Build history of the part. All positions in model axes, mm. A direction names the side the tool comes from. Round coordinates to 2 decimals unless told otherwise and drop trailing zeros. Loops run counter-clockwise (first coordinate to the right, second up) from the corner with the lowest first, then second, coordinate; pieces in that order, holes last. Notation, with made-up numbers: (-33.5, -16) - (-22.5, -16) arc R10 cw to (-22.5, 1) - close; hole circle Ø7 at (9, 10.5). An arc over 180 degrees is marked (long way). Use one line per item in the form item = value. Start each with the question number.
Q1. Pin check, flat tips, straight feed: pin 1 (3 mm diameter, centred on y = 4.5, z = -0.5, fed in from +X); pin 2 (4.5 mm diameter, centred on x = 5.5, z = 2, fed in from +Y); pin 3 (1.5 mm diameter, centred on x = 9.5, y = 6, fed in from -Z); pin 4 (1.8 mm diameter, centred on x = 5.5, y = 4, fed in from +Z). Stop position of each tip, or through.
Q2. Saw through at C-C (y = 2). Give the cut face in (x, z).
Q3. Saw through at A-A (x = 6). Give the cut face in (y, z) (3 decimals), then the cut area to 3 significant figures.
Q4. Saw through at B-B (z = 3). Give the cut face in (x, y) (3 decimals).
Q5. Drill centre lines: line 1 (Y direction, x = 38, z = 3) (3 decimals); line 2 (Y direction, x = 6, z = 5.3); line 3 (X direction, y = 10.5, z = -5). Where is each one in solid material? Low to high.
Q6. Mould opens along X. For faces 6 (the face through (0, 4, 3)), 7 (the face through (38, 6.5, 0.15)), 8 (the face through (6, 2, 4)), 9 (the face through (35, 4.6, 5)) say: released by +X, released by -X, zero draft, split by the parting line, or undercut.
Q7. Saw through at D-D (z = 5). Give the cut face in (x, y), then the cut area to 3 significant figures.
Q8. 3-axis set-ups, long thin cutter, end or side, ignore diameter. For faces 1 (the face through (6, 8.85, 3)), 2 (the face through (38, 8.85, 3)), 3 (the face through (8, 5, 0.15)), 4 (the face through (22, 5, 6)), 5 (the face through (40, 5, 4)): which of +Z, -Z, +X, -X, +Y, -Y reach the whole face in a straight line?
Autodesk Inventor part; units mm, degrees
ref_plane "YZ Plane" through (0, 0, 0) normal (1, 0, 0) x (0, 1, 0)
ref_plane "XZ Plane" through (0, 0, 0) normal (0, 1, 0) x (-1, 0, 0)
ref_plane "XY Plane" through (0, 0, 0) normal (0, 0, 1) x (1, 0, 0)
sketch "Sketch1" plane through (0, 0, 0) normal (0, 0, 1) x (1, 0, 0)
  line L0 (0, 0) -> (44, 0)
  line L1 (44, 0) -> (44, 8.85)
  line L2 (31.85, 12) -> (12.15, 12)
  line L3 (0, 8.85) -> (0, 0)
  line L4 (12.15, 12) -> (12.15, 8.85)
  line L5 (12.15, 8.85) -> (0, 8.85)
  line L6 (31.85, 12) -> (31.85, 8.85)
  line L7 (31.85, 8.85) -> (44, 8.85)
  dimension "d6" = 44
  dimension "d7" = 3.15
  dimension "d8" = 3.15
  dimension "d9" = 12.15
  dimension "d10" = 12.15
  dimension "d11" = 8.85
  dimension "d12" = 8.85
  dimension "d13" = 12
extrude "Extrusion1" add sketch "Sketch1" along normal blind 6
sketch "Sketch2" plane through (0, 0, 0) normal (0, 0, -1) x (-1, 0, 0)
  line L0 (-31.85, 12) -> (-12.15, 12)
  line L1 (0, 0) -> (-44, 0)
  line L2 (-31.85, 12) -> (-12, 12)
  line L3 (-12, 12) -> (-12, 0)
  line L4 (-12, 0) -> (-31.85, 0)
  line L5 (-31.85, 0) -> (-31.85, 12)
extrude "Extrusion2" add sketch "Sketch2" along normal blind 6
sketch "Sketch3" plane through (0, 0, 0) normal (0, 0, -1) x (-1, 0, 0)
  circle A0 centre (-6, 4.35) radius 1.725
  line L0 (-12, 8.85) -> (0, 8.85)
  line L1 (0, 8.85) -> (0, 0)
  circle A1 centre (-38, 4.5) radius 1.725
  line L2 (-31.85, 0) -> (-44, 0)
  line L3 (-44, 0) -> (-44, 8.85)
  point P0 (-12, 9)
  dimension "d18" = 3.45
  dimension "d19" = 4.5
  dimension "d20" = 6
  dimension "d21" = 3.45
  dimension "d22" = 4.5
  dimension "d23" = 6
extrude "Extrusion3" cut sketch "Sketch3" against normal blind 4
sketch "Sketch4" plane through (0, 0, 6) normal (0, 0, 1) x (1, 0, 0)
  circle A0 centre (6, 4.35) radius 3
  line L0 (12.15, 8.85) -> (0, 8.85)
  line L1 (0, 8.85) -> (0, 0)
  circle A1 centre (38, 4.5) radius 1.725
  circle A2 centre (38, 4.5) radius 3
  dimension "d26" = 6
  dimension "d27" = 4.5
  dimension "d28" = 6
  dimension "d29" = 6
extrude "Extrusion4" cut sketch "Sketch4" against normal blind 2 contours A0 | A1 | A2
sketch "Sketch5" plane through (31.85, 0, 0) normal (0, -1, 0) x (1, 0, 0)
  point P0 (-31.85, 0)
sketch "Sketch6" plane through (0, 0, 0) normal (0, 0, -1) x (-1, 0, 0)
  line L0 (0, 0) -> (-44, 0)
  line L1 (-12.15, 8.85) -> (0, 8.85)
  line L2 (0, 0) -> (0, 8.85)
  line L3 (-12.15, 8.85) -> (-12, 8.85)
  line L4 (0, 8.85) -> (-12, 8.85)
  line L5 (-12, 0) -> (-12, 12)
  line L6 (-12, 8.85) -> (-12, 0)
  line L7 (-12, 0) -> (0, 0)
  line L8 (-44, 0) -> (-44, 8.85)
  line L9 (-44, 0) -> (-31.85, 0)
  line L10 (-31.85, 0) -> (-31.85, 8.85)
  line L11 (-31.85, 0) -> (-31.85, 8.85)
  line L12 (-31.85, 8.85) -> (-44, 8.85)
  line L13 (-44, 8.85) -> (-44, 0)
  dimension "d33" = 12.15
extrude "Extrusion5" cut sketch "Sketch6" against normal blind 0.15
sketch "Sketch7" plane through (12, 8.85, 0) normal (-1, 0, 0) x (0, 0, 1)
  line L0 (0, 3.15) -> (0, 0)
  line L1 (0, 3.15) -> (0, 0)
  line L2 (0.15, 0) -> (6, 0)
  line L3 (0, 0) -> (0.15, 0)
  line L4 (0.15, 0) -> (0.15, -8.85)
  line L5 (0.15, 0) -> (0.15, -8.85)
  line L6 (0.15, -8.85) -> (-6, -8.85)
  line L7 (0.15, -8.85) -> (-6, -8.85)
  line L8 (-6, -8.85) -> (-6, 3.15)
  line L9 (0, 3.15) -> (6, 3.15)
  line L10 (-6, 3.15) -> (0, 3.15)
  point P0 (0, -8.85)
sketch "Sketch8" plane through (12.15, 12, 6) normal (0, 1, 0) x (1, 0, 0)
  line L0 (0, 6) -> (0, 0)
  line L1 (19.7, 12) -> (-0.15, 12)
  line L2 (0, 6) -> (-0.15, 6)
  line L3 (-0.15, 6) -> (-0.15, 12)
  line L4 (-0.15, 12) -> (0, 12)
  line L5 (0, 12) -> (0, 6)
  point P0 (-12.15, 6)
extrude "Extrusion6" cut sketch "Sketch7" against normal blind 0.15
fillet "Fillet2" radius 1.5 2 edges at (22, 12, 6) (22, 12, -6)
sketch "Sketch9" plane through (0, 0, 6) normal (0, 0, 1) x (1, 0, 0)
  point P0 (0, 0)
equation "\"d8\" = d7"
equation "\"d10\" = d9"
equation "\"d12\" = d11"
properties part number "beam44mmVer2"
Report:
q1.pin_1 = 44
q1.pin_2 = 8.85
q1.pin_3 = 0.15
q1.pin_4 = through
q2.outline = (0, 0.15) - (12.15, 0.15) - (12.15, -6) - (31.85, -6) - (31.85, 0.15) - (44, 0.15) - (44, 6) - (39.66, 6) - (39.66, 4) - (36.34, 4) - (36.34, 6) - (7.86, 6) - (7.86, 4) - (4.14, 4) - (4.14, 6) - (0, 6) - close
q3.outline = (0, 0.15) - (2.625, 0.15) - (2.625, 4) - (1.35, 4) - (1.35, 6) - (0, 6) - close; (6.075, 0.15) - (8.85, 0.15) - (8.85, 6) - (7.35, 6) - (7.35, 4) - (6.075, 4) - close
q3.area = 26.5 mm²
q4.outline = (0, 0) - (44, 0) - (44, 8.85) - (31.85, 8.85) - (31.85, 12) - (12.15, 12) - (12.15, 8.85) - (0, 8.85) - close; hole circle Ø3.45 at (6, 4.35); hole circle Ø3.45 at (38, 4.5)
q5.line_1 = 0 to 2.775, 6.225 to 8.85
q5.line_2 = 0 to 1.35, 7.35 to 8.85
q5.line_3 = 12.15 to 31.85
q6.face_6 = released by -X
q6.face_7 = zero draft
q6.face_8 = undercut
q6.face_9 = undercut
q7.outline = (0, 0) - (44, 0) - (44, 8.85) - (31.85, 8.85) - (31.85, 11.91) - (12.15, 11.91) - (12.15, 8.85) - (0, 8.85) - close; hole circle Ø6 at (6, 4.35); hole circle Ø6 at (38, 4.5)
q7.area = 393 mm²
q8.face_1 = +Z, -Z, -X, +Y
q8.face_2 = +Z, -Z, +X, +Y
q8.face_3 = -Z, -X, +Y, -Y
q8.face_4 = +Z, +X, -X, +Y, -Y
q8.face_5 = +Z
